Design review of the part shown in the three views and the two pictorial views. Dimensions are in mm from the part's minimum x, y and z. A direction names the side the tool comes from. Round coordinates to 2 decimals unless told otherwise and drop trailing zeros. Loops run counter-clockwise (first coordinate to the right, second up) from the corner with the lowest first, then second, coordinate; pieces in that order, holes last. Notation, with made-up numbers: (-4.5, 73) - (37.5, 73) arc R15 cw to (37.5, 79) - close; hole circle Ø11 at (-2, 20). An arc over 180 degrees is marked (long way). Return JSON: item names as keys, results as strings. Group by question number.
(1) We need section A-A, the plane y = 57.2. Write out the cut boundary in (x, z).
(2) Wall thickness on L1, parallel to Z at x = 9, y = 16; L2, parallel to Y at x = 9, z = 16.5: over which ranges is each line inside the solid? List them lowest first. Write a range as [from, to].
(3) We need section C-C, the plane z = 1. Write out the cut boundary in (x, y), and give its area (3 significant figures).
(4) For the marked faces 1 and 2, list the 3-axis set-ups (+Z, -Z, +X, -X, +Y, -Y) from which the entire face can be reached by the end or side of a thin tool; tool diameter is ignored.
(5) The part is to be moulded in two halves that separate along X. For the marked faces 3, 4, 5 and 6, say which applies: pulls with the +X half, pulls with the -X half, needs draft (parallel to the pull), parting line crosses it, or undercut.
(6) Clearance check with a flat-ended pin moving along its axis: pin 1 (4 mm diameter, centred on x = 12, z = 12, fed in from -Y). State where the tip first meets the part, or that it passes through.
(7) We need section B-B, the plane x = 12.75. Write out the cut boundary in (y, z) (1 decimal), and give its area (3 significant figures).
(8) We need section D-D, the plane y = 26.5. Write out the cut boundary in (x, z), and give its area (3 significant figures).
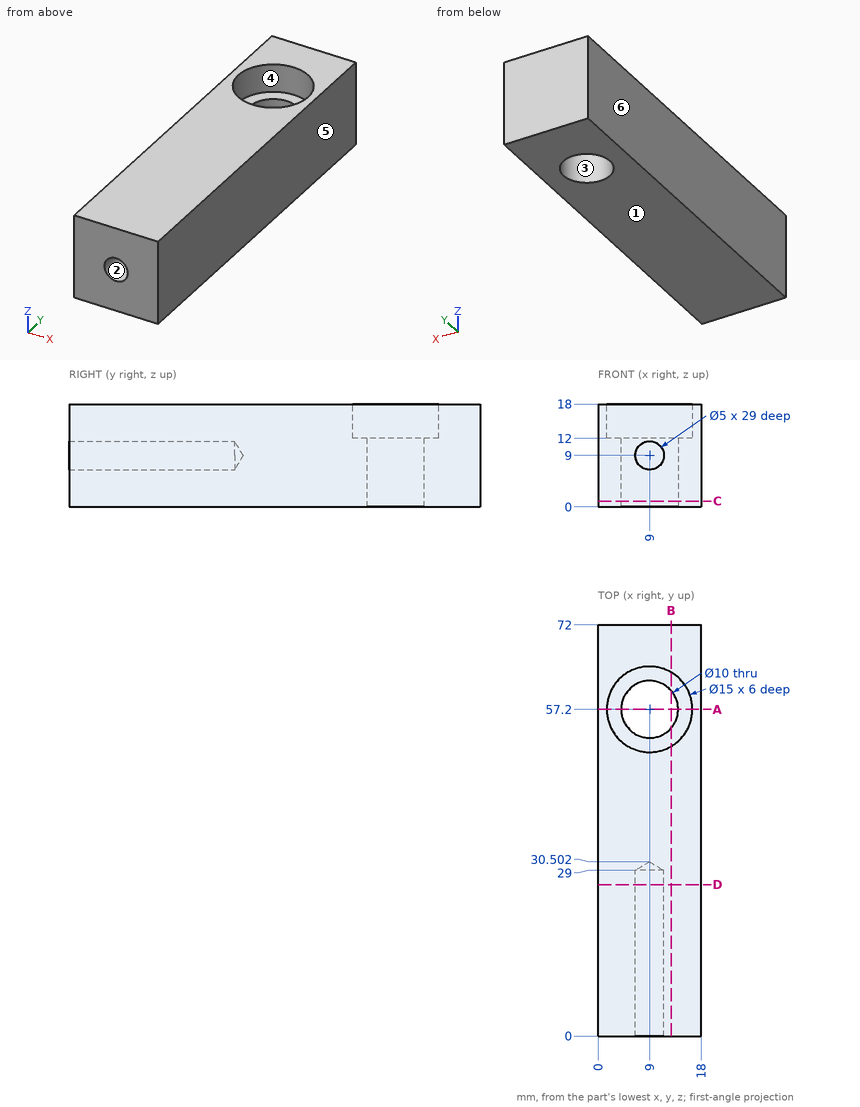
Solutions:
{
 "1": {"outline": "(0, 0) - (4, 0) - (4, 12) - (1.5, 12) - (1.5, 18) - (0, 18) - close; (14, 0) - (18, 0) - (18, 18) - (16.5, 18) - (16.5, 12) - (14, 12) - close"},
 "2": {"L1": "[0, 6.5], [11.5, 18]", "L2": "[0, 49.7], [64.7, 72]"},
 "3": {"outline": "(0, 0) - (18, 0) - (18, 72) - (0, 72) - close; hole circle Ø10 at (9, 57.2)", "area": "1,220 mm^2"},
 "4": {"face 1": "-Z, +X, -X, +Y, -Y", "face 2": "-Y"},
 "5": {"face 3": "undercut", "face 4": "undercut", "face 5": "pulls with the +X half", "face 6": "pulls with the -X half"},
 "6": {"pin 1": "y = 0"},
 "7": {"outline": "(0, 0) - (53.9, 0) - (53.9, 12) - (50.7, 12) - (50.7, 18) - (0, 18) - close; (60.5, 0) - (72, 0) - (72, 18) - (63.7, 18) - (63.7, 12) - (60.5, 12) - close", "area": "1,140 mm^2"},
 "8": {"outline": "(0, 0) - (18, 0) - (18, 18) - (0, 18) - close; hole circle Ø5 at (9, 9)", "area": "304 mm^2"}
}
